```python
from build123d import *

# Parameters (mm, degrees)
SKETCH1_R           = 16.8
BOSS_EXTRUDE1_DEPTH = 16
SKETCH2_R           = 4
CUT_EXTRUDE1_DEPTH  = 29.644022064
SKETCH3_R           = 1
CUT_EXTRUDE2_DEPTH  = 5
SKETCH4_R           = 1.5
CUT_EXTRUDE3_DEPTH  = 5


with BuildPart() as part:
    # Sketch1 → Boss-Extrude1 (new body)
    with BuildSketch(Plane(origin=(0, 0, 0), x_dir=(1, 0, 0), z_dir=(0, 1, 0))):
        with Locations(Location((0, 0, 0), (0, 0, 270))):
            Circle(SKETCH1_R)
    extrude(amount=BOSS_EXTRUDE1_DEPTH)

    # Sketch2 → Cut-Extrude1 (cut, through all)
    with BuildSketch(Plane(origin=(0, 16, 0), x_dir=(1, 0, 0), z_dir=(0, 1, 0))):
        with Locations(Location((0, 0, 0), (0, 0, 270))):
            Circle(SKETCH2_R)
    extrude(amount=-CUT_EXTRUDE1_DEPTH, mode=Mode.SUBTRACT)

    # Sketch3 → Cut-Extrude2 (cut)
    with BuildSketch(Plane(origin=(0, 16, 0), x_dir=(1, 0, 0), z_dir=(0, 1, 0))):
        with Locations(Location((0, 7.5, 0), (0, 0, 270))):
            Circle(SKETCH3_R)
        with Locations(Location((0, -7.5, 0), (0, 0, 270))):
            Circle(SKETCH3_R)
    extrude(amount=-CUT_EXTRUDE2_DEPTH, mode=Mode.SUBTRACT)

    # Sketch4 → Cut-Extrude3 (cut)
    with BuildSketch(Plane.XZ):
        with Locations(Location((0, 11.25, 0), (0, 0, 270))):
            Circle(SKETCH4_R)
        with Locations(Location((11.25, 0, 0), (0, 0, 270))):
            Circle(SKETCH4_R)
        with Locations(Location((0, -11.25, 0), (0, 0, 270))):
            Circle(SKETCH4_R)
        with Locations(Location((-11.25, 0, 0), (0, 0, 270))):
            Circle(SKETCH4_R)
    extrude(amount=-CUT_EXTRUDE3_DEPTH, mode=Mode.SUBTRACT)


solid = part.part
```
CAD build for the part. Positions are in the model's coordinates, mm. A direction names the side the tool comes from. Round coordinates to 2 decimals unless told otherwise and drop trailing zeros. Order: outer loops, then holes, each group sorted by start corner. A loop starts at its lowest first (then second) coordinate and runs counter-clockwise, first axis right, second up.
Q1. Slice it at D-D (y = 12.75). Write the cut outline in (x, z).
Q2. Slice it at B-B (x = -11.25). Write the cut outline in (y, z), and give its area (3 significant figures).
Q3. Which spindle directions (+Z, -Z, +X, -X, +Y, -Y) get a long thin tool onto all of the face, cutting with end or side? Do faces 1 (the flat face through (11, 5, 0)), 2 (the cylindrical face through (-3.905, 8.112, -0.867)), 3 (the flat face through (0, 11, 7)). Say none if no direction does.
Q4. Slice it at C-C (z = 7.5). Write the cut outline in (x, y).
Q5. Two-plate mould, pull along X, no slides. Class faces 4 (the cylindrical face through (-0.6, 13.5, -8.3)), 5 (the flat face through (-3, 16, 3)), 6 (the cylindrical face through (5.046, 7.888, 16.024)): pulls with the +X half, pulls with the -X half, needs draft (parallel to the pull), parting line crosses it, or undercut.
Q6. Slice it at A-A (y = 2). Write the cut outline in (x, z).
Q7. Wall check: L1, parallel to X at y = 6.5, z = 0; L2, parallel to X at y = 14.3, z = -7.5; L3, parallel to Z at x = 11.5, y = 11.5. Give the ranges that are in metal, low to high.
Q8. Drop flat-ended pins along their axis: pin 1 (1 mm diameter, centred on x = -0.5, z = 8, fed in from +Y); pin 2 (5 mm diameter, centred on x = -5.5, y = 9, fed in from +Z); pin 3 (0.9 mm diameter, centred on x = -11.5, z = 0, fed in from -Y); pin 4 (8 mm diameter, centred on y = 5.5, z = 10, fed in from +X). Give the stop position or say it passes through.
Results below:
1. outline: circle Ø33.6 at (0, 0); hole circle Ø8 at (0, 0); hole circle Ø2 at (0, -7.5); hole circle Ø2 at (0, 7.5)
2. outline: (0, -12.48) - (16, -12.48) - (16, 12.48) - (0, 12.48) - (0, 1.5) - (5, 1.5) - (5, -1.5) - (0, -1.5) - close
2. area: 384 mm2
3. face 1: -Y
3. face 2: +Y, -Y
3. face 3: +Y
4. outline: (-15.03, 0) - (15.03, 0) - (15.03, 16) - (1, 16) - (1, 11) - (-1, 11) - (-1, 16) - (-15.03, 16) - close
5. face 4: undercut
5. face 5: needs draft
5. face 6: parting line crosses it
6. outline: circle Ø33.6 at (0, 0); hole circle Ø3 at (-11.25, 0); hole circle Ø8 at (0, 0); hole circle Ø3 at (0, -11.25); hole circle Ø3 at (0, 11.25); hole circle Ø3 at (11.25, 0)
7. L1: x = -16.8 to -4, 4 to 16.8
7. L2: x = -15.03 to -1, 1 to 15.03
7. L3: z = -12.25 to 12.25
8. pin 1: stops at y = 16
8. pin 2: stops at z = 16.53
8. pin 3: stops at y = 5
8. pin 4: stops at x = 15.69
